from build123d import *

# Parameters (mm, degrees)
SKETCH1_R          = 2.9945
EXTRUDE1_DEPTH     = 19.7
SKETCH2_R          = 10.975
EXTRUDE2_DEPTH     = 2.4
SKETCH3_R          = 19.925
EXTRUDE3_DEPTH     = 70
SKETCH4_R          = 2.9945
EXTRUDE4_DEPTH     = 13.5
SKETCH5_R          = 1.5
CUT_EXTRUDE1_DEPTH = 8
SKETCH6_R          = 0.8
CUT_EXTRUDE2_DEPTH = 4
CUT_EXTRUDE3_START = -2.5
CUT_EXTRUDE3_DEPTH = 2.5


with BuildPart() as part:
    # Sketch1 → Extrude1 (new body)
    with BuildSketch(Plane(origin=(0, 0, 0), x_dir=(0, 0, -1), z_dir=(1, 0, 0))):
        Circle(SKETCH1_R)
    extrude(amount=EXTRUDE1_DEPTH)

    # Sketch2 → Extrude2 (add)
    with BuildSketch(Plane(origin=(19.7, 0, 0), x_dir=(0, 0, -1), z_dir=(1, 0, 0))):
        Circle(SKETCH2_R)
    extrude(amount=-EXTRUDE2_DEPTH)

    # Sketch3 → Extrude3 (add)
    with BuildSketch(Plane(origin=(19.7, 0, 0), x_dir=(0, 0, -1), z_dir=(1, 0, 0))):
        Circle(SKETCH3_R)
    extrude(amount=EXTRUDE3_DEPTH)

    # Sketch4 → Extrude4 (add)
    with BuildSketch(Plane(origin=(89.7, 0, 0), x_dir=(0, 0, -1), z_dir=(1, 0, 0))):
        Circle(SKETCH4_R)
    extrude(amount=EXTRUDE4_DEPTH)

    # Sketch5 → Cut-Extrude1 (cut)
    with BuildSketch(Plane.ZY.offset(-19.7)):
        with Locations((11.313708499, 11.313708499)):
            Circle(SKETCH5_R)
        with Locations((11.313708499, -11.313708499)):
            Circle(SKETCH5_R)
        with Locations((-11.313708499, -11.313708499)):
            Circle(SKETCH5_R)
        with Locations((-11.313708499, 11.313708499)):
            Circle(SKETCH5_R)
    extrude(amount=-CUT_EXTRUDE1_DEPTH, mode=Mode.SUBTRACT)

    # Sketch6 → Cut-Extrude2 (cut)
    with BuildSketch(Plane(origin=(89.7, 0, 0), x_dir=(0, 0, -1), z_dir=(1, 0, 0))):
        with Locations((0, 10.45)):
            Circle(SKETCH6_R)
        with Locations((9.04996547, -5.225)):
            Circle(SKETCH6_R)
        with Locations((-9.04996547, -5.225)):
            Circle(SKETCH6_R)
    extrude(amount=-CUT_EXTRUDE2_DEPTH, mode=Mode.SUBTRACT)

    # Sketch7 → Cut-Extrude3 (cut)
    with BuildSketch(Plane(origin=(89.7, 0, 0), x_dir=(0, 0, -1), z_dir=(1, 0, 0)).offset(CUT_EXTRUDE3_START)):
        with BuildLine():
            Line((-7, -15.925), (7, -15.925))
            Line((7, -15.925), (7, -18.654908871))
            ThreePointArc((7, -18.654908871), (0, -19.925), (-7, -18.654908871))
            Line((-7, -18.654908871), (-7, -15.925))
        make_face()
    extrude(amount=CUT_EXTRUDE3_DEPTH, mode=Mode.SUBTRACT)


solid = part.part
The model under review builds one solid part; all positions refer to its coordinate system, in mm. A direction names the side the tool comes from. Give positions to 0.01 mm unless a question says otherwise; leave off trailing zeros. Order: outer loops, then holes, each group sorted by start corner. A loop starts at its lowest first (then second) coordinate and runs counter-clockwise, first axis right, second up. Notation, with made-up numbers: M 21.25,-13.75 L 52.25,-13.75 A23 ccw 52.25,10.25 Z; hole C -25.5,12 d3. An arc over 180 degrees is marked long. Use one line per item in the form item = value. Start each with the question number.
Item 1: We need section D-D on z = 5. Give the boundary of the cut face in (x, y) (3 decimals).
Item 2: The part is to be moulded in two halves that separate along Z. For faces 1 (the cylindrical face through (23.644, -10.863, -9.883)), 2 (the flat face through (0, 0, 0)), 3 (the cylindrical face through (18.52, 10.88, 1.43)), say which applies: pulls with the +Z half, pulls with the -Z half, needs draft (parallel to the pull), parting line crosses it, or undercut.
Item 3: We need section A-A on y = 0. Give the boundary of the cut face in (x, z) (1 decimal), plus the area to 3 significant figures.
Item 4: We need section B-B on x = 26. Give the boundary of the cut face in (y, z) (3 decimals).
Item 5: For faces 4 (the flat face through (88, -17, 7)), 5 (the cylindrical face through (54, 6, -19)), 6 (the cylindrical face through (23.644, -11.248, 9.815)), list the 3-axis set-ups (+Z, -Z, +X, -X, +Y, -Y) from which the entire face can be reached by the end or side of a thin tool; tool diameter is ignored.
Item 6: We need section C-C on x = 74.5. Give the boundary of the cut face in (y, z) (3 decimals).
Item 7: To check wall thickness, follow line 1 along X through (y, z) = (14, 2.5); line 2 along X through (y, z) = (4, -10); line 3 along Z through (x, y) = (53.5, 8). State the ranges of each line that lie inside material, in increasing order. Write a range as from..to.
Item 8: Insertion check: pin 1 Ø1.8 at (y, z) = (-11.31, -11.31) entering from -X; pin 2 Ø1.3 at (y, z) = (-5.5, -9.5) entering from +X; pin 3 Ø4 at (x, z) = (16.5, 3) entering from -Y. Each pin has a flat end and moves straight along its axis. Give the tip position at first contact, or say it passes through.
Completed:
q1.outline = M 17.3,-9.77 L 19.7,-9.77 L 19.7,-19.287 L 87.2,-19.287 L 87.2,-15.925 L 89.7,-15.925 L 89.7,19.287 L 19.7,19.287 L 19.7,9.77 L 17.3,9.77 Z
q2.face_1 = undercut
q2.face_2 = needs draft
q2.face_3 = parting line crosses it
q3.outline = M 0,-3 L 17.3,-3 L 17.3,-11 L 19.7,-11 L 19.7,-19.9 L 89.7,-19.9 L 89.7,-3 L 103.2,-3 L 103.2,3 L 89.7,3 L 89.7,19.9 L 19.7,19.9 L 19.7,11 L 17.3,11 L 17.3,3 L 0,3 Z
q3.area = 3,030 mm²
q4.outline = C 0,0 d39.85; hole C -11.314,-11.314 d3; hole C -11.314,11.314 d3; hole C 11.314,-11.314 d3; hole C 11.314,11.314 d3
q5.face_4 = +X, -Y
q5.face_5 = +X, -X
q5.face_6 = -X
q6.outline = C 0,0 d39.85
q7.line_1 = 19.7..89.7
q7.line_2 = 17.3..89.7
q7.line_3 = -18.25..18.25
q8.pin_1 = 27.7
q8.pin_2 = 89.7
q8.pin_3 = -10.91
